Source: three-view drawing plus pictorial views. Frame: mm from the lowest corner of the part. Coordinates: 2 decimals unless noted, no trailing zeros. Loops run counter-clockwise (first coordinate to the right, second up) from the corner with the lowest first, then second, coordinate; pieces in that order, holes last. Notation, with made-up numbers: (29.5, 84.5) - (65.5, 84.5) arc R22 ccw to (65.5, 92.5) - close; hole circle Ø6 at (4, 9). An arc over 180 degrees is marked (long way). Return JSON: item names as keys, results as strings.
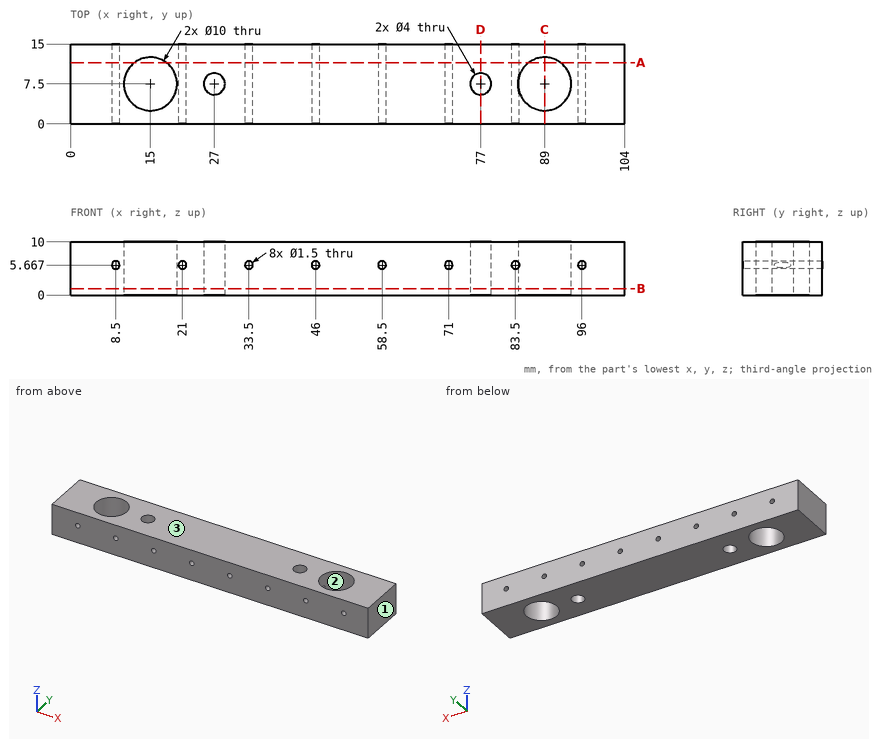
Item 1: Ray query, probe 1 along Z at (x, y) = (83.5, 8.75); probe 2 along Y at (x, z) = (89, 5.5); probe 3 along X at (y, z) = (9, 7.5) (1 decimal). Return the intervals inside material, ascending. Write a range as from..to.
Worked out:
{"probe 1": "0..4.92, 6.42..10", "probe 2": "0..2.5, 12.5..15", "probe 3": "0..10.2, 19.8..25.7, 28.3..75.7, 78.3..84.2, 93.8..104"}
Item 2: Section query A-A, the plane y = 11.5. Count the separate pieces of the cut face and the enclosed holes in it, and give its area (3 significant figures).
Worked out:
{"separate pieces": "3", "enclosed holes": "8", "area": "906 mm^2"}
Item 3: Mould query, pull axis X, two halves, no side actions, for the marked faces 1, 2 and 3. Classes: +X half, -X half, draft (parallel to the pull), parting line (faces both ways), or undercut.
Worked out:
{"face 1": "+X half", "face 2": "undercut", "face 3": "draft"}
Item 4: Section query C-C, the plane x = 89. Return loops of the section in (y, z).
Worked out:
{"outline": "(0, 0) - (2.5, 0) - (2.5, 10) - (0, 10) - close; (12.5, 0) - (15, 0) - (15, 10) - (12.5, 10) - close"}
Item 5: Section query D-D, the plane x = 77. Return loops of the section in (y, z), and give its area (3 significant figures).
Worked out:
{"outline": "(0, 0) - (5.5, 0) - (5.5, 10) - (0, 10) - close; (9.5, 0) - (15, 0) - (15, 10) - (9.5, 10) - close", "area": "110 mm^2"}
Item 6: Section query B-B, the plane z = 1.25. Return loops of the section in (x, y).
Worked out:
{"outline": "(0, 0) - (104, 0) - (104, 15) - (0, 15) - close; hole circle Ø10 at (15, 7.5); hole circle Ø4 at (27, 7.5); hole circle Ø4 at (77, 7.5); hole circle Ø10 at (89, 7.5)"}
